from build123d import *

# Parameters (mm, degrees)
SKETCH1_W               = 35
SKETCH1_H               = 25
BOSS_EXTRUDE1_DEPTH     = 8.5
SKETCH3_W               = 32
SKETCH3_H               = 25
CUT_EXTRUDE1_DEPTH      = 7
FILLET1_R               = 1
CHAMFER1_SIZE           = 2.5
SKETCH4_R               = 1.25
CUT_EXTRUDE2_DEPTH      = 35
SKETCH5_R               = 3
BOSS_EXTRUDE3_DEPTH     = 2.5
SKETCH7_R               = 4
SKETCH7_R_2             = 1.25
CUT_EXTRUDE3_DEPTH      = 2.5
CUT_EXTRUDE3_DEPTH_BACK = 1.5


with BuildPart() as part:
    # Sketch1 → Boss-Extrude1 (new body)
    with BuildSketch(Plane.XY):
        with Locations((17.5, 12.5)):
            Rectangle(SKETCH1_W, SKETCH1_H)
    extrude(amount=BOSS_EXTRUDE1_DEPTH)

    # Sketch3 → Cut-Extrude1 (cut)
    with BuildSketch(Plane.XY.offset(8.5)):
        with Locations((17.5, 12.5)):
            Rectangle(SKETCH3_W, SKETCH3_H)
    extrude(amount=-CUT_EXTRUDE1_DEPTH, mode=Mode.SUBTRACT)

    # Fillet1
    fillet1_edges = [part.edges().sort_by_distance(p)[0] for p in [
        (0, 12.5, 0),
        (35, 12.5, 0),
    ]]
    fillet(fillet1_edges, radius=FILLET1_R)

    # Chamfer1
    chamfer1_edges = [part.edges().sort_by_distance(p)[0] for p in [
        (0.75, 0, 8.5),
        (0.75, 25, 8.5),
        (34.25, 0, 8.5),
        (34.25, 25, 8.5),
    ]]
    chamfer(chamfer1_edges, length=CHAMFER1_SIZE)

    # Sketch4 → Cut-Extrude2 (cut)
    with BuildSketch(Plane.ZY):
        with Locations((6, 20)):
            Circle(SKETCH4_R)
        with Locations((6, 4)):
            Circle(SKETCH4_R)
    extrude(amount=-CUT_EXTRUDE2_DEPTH, mode=Mode.SUBTRACT)

    # Sketch5 → Boss-Extrude3 (add)
    with BuildSketch(Plane.XY.offset(1.5)):
        with Locations((9.5, 4.5)):
            Circle(SKETCH5_R)
        with Locations((25.5, 4.5)):
            Circle(SKETCH5_R)
        with Locations((25.499999171, 20.5)):
            Circle(SKETCH5_R)
        with Locations((9.499999171, 20.5)):
            Circle(SKETCH5_R)
    extrude(amount=BOSS_EXTRUDE3_DEPTH)

    # Sketch7 → Cut-Extrude3 (cut, two sides)
    with BuildSketch(Plane.XY.offset(1.5)) as cut_extrude3_sk:
        with Locations((17.5, 12.5)):
            Circle(SKETCH7_R)
        with Locations((9.5, 4.5)):
            Circle(SKETCH7_R_2)
        with Locations((17.5, 4.5)):
            Circle(SKETCH7_R_2)
        with Locations((25.5, 4.5)):
            Circle(SKETCH7_R_2)
        with Locations((25.5, 12.5)):
            Circle(SKETCH7_R_2)
        with Locations((17.5, 20.5)):
            Circle(SKETCH7_R_2)
        with Locations((25.5, 20.5)):
            Circle(SKETCH7_R_2)
        with Locations((9.5, 12.5)):
            Circle(SKETCH7_R_2)
        with Locations((9.5, 20.5)):
            Circle(SKETCH7_R_2)
    extrude(amount=CUT_EXTRUDE3_DEPTH, mode=Mode.SUBTRACT)
    extrude(cut_extrude3_sk.sketch, amount=-CUT_EXTRUDE3_DEPTH_BACK, mode=Mode.SUBTRACT)


solid = part.part
Geometry check sheet. Reference: the model listing, model coordinates, mm. A direction names the side the tool comes from. Coordinates: 2 decimals unless noted, no trailing zeros. Order: outer loops, then holes, each group sorted by start corner. A loop starts at its lowest first (then second) coordinate and runs counter-clockwise, first axis right, second up. Notation, with made-up numbers: (27.25, -29) -> (42.25, -29) arc R25 cw to (42.25, -11) -> close; hole circle Ø5 at (-0.5, 56.5). An arc over 180 degrees is marked (long way). Use a Markdown table: item, result. Add a question column.
1. Go/stop test with flat-tipped pins: pin 1 Ø2 at (y, z) = (20, 6) entering from +X; pin 2 Ø5 at (x, y) = (24.5, 5) entering from +Z; pin 3 Ø3 at (x, y) = (17.5, 4.5) entering from +Z; pin 4 Ø3 at (x, z) = (21.5, 4) entering from +Y. Record where each tip stops, or that it passes through.
2. Cross-section at D-D (y = 9.25). Enter the section's corners in (x, z).
3. Set-up check for faces 5 (the face through (1, 24, 7)), 6 (the face through (28.27, 19.35, 2.73)), 7 (the face through (33.5, 12, 5)): record each of +Z, -Z, +X, -X, +Y, -Y from which the full face is reachable in a straight line by a thin tool's end or side.
4. Cross-section at B-B (x = 9.5). Enter the section's corners in (y, z).
5. Cross-section at C-C (y = 11.75). Enter the section's corners in (x, z), and give its area (3 significant figures).
6. Cross-section at A-A (z = 3.5). Give the number of separate pieces and of enclosed holes in the cut face, and give its area (3 significant figures).
7. Material ranges on L1, parallel to Y at x = 25.5, z = 0.4; L2, parallel to Y at x = 17.5, z = 0.6; L3, parallel to X at y = 2.5, z = 6.75, recorded low to high.
8. Mould release check, pull along X, two halves, no side actions. Record for faces 1 (the face through (27, 5, 4)), 2 (the face through (0.285, 12.675, 0.301)), 3 (the face through (25, 19, 4)), 4 (the face through (34, 24, 7)): pulls with the +X half, pulls with the -X half, needs draft (parallel to the pull), parting line crosses it, or undercut.
Filled sheet:
| question | item | result |
|---|---|---|
| 1 | pin 1 | through |
| 1 | pin 2 | z = 4 |
| 1 | pin 3 | z = 1.5 |
| 1 | pin 4 | y = 22.16 |
| 2 | outline | (0, 1) arc R1 ccw to (1, 0) -> (15.17, 0) -> (15.17, 1.5) -> (1.5, 1.5) -> (1.5, 8.5) -> (0, 8.5) -> close; (19.83, 0) -> (34, 0) arc R1 ccw to (35, 1) -> (35, 8.5) -> (33.5, 8.5) -> (33.5, 1.5) -> (19.83, 1.5) -> close |
| 3 | face 5 | +Z, +X, -X, +Y |
| 3 | face 6 | +Z |
| 3 | face 7 | +Z, +Y, -Y |
| 4 | outline | (0, 0) -> (3.25, 0) -> (3.25, 4) -> (1.5, 4) -> (1.5, 1.5) -> (0, 1.5) -> close; (5.75, 0) -> (11.25, 0) -> (11.25, 1.5) -> (7.5, 1.5) -> (7.5, 4) -> (5.75, 4) -> close; (13.75, 0) -> (19.25, 0) -> (19.25, 4) -> (17.5, 4) -> (17.5, 1.5) -> (13.75, 1.5) -> close; (21.75, 0) -> (25, 0) -> (25, 1.5) -> (23.5, 1.5) -> (23.5, 4) -> (21.75, 4) -> close |
| 5 | outline | (0, 1) arc R1 ccw to (1, 0) -> (8.5, 0) -> (8.5, 1.5) -> (1.5, 1.5) -> (1.5, 8.5) -> (0, 8.5) -> close; (10.5, 0) -> (13.57, 0) -> (13.57, 1.5) -> (10.5, 1.5) -> close; (21.43, 0) -> (24.5, 0) -> (24.5, 1.5) -> (21.43, 1.5) -> close; (26.5, 0) -> (34, 0) arc R1 ccw to (35, 1) -> (35, 8.5) -> (33.5, 8.5) -> (33.5, 1.5) -> (26.5, 1.5) -> close |
| 5 | area | 55.3 mm2 |
| 6 | separate pieces | 6 |
| 6 | enclosed holes | 4 |
| 6 | area | 168 mm2 |
| 7 | L1 | 0 to 3.25, 5.75 to 11.25, 13.75 to 19.25, 21.75 to 25 |
| 7 | L2 | 0 to 3.25, 5.75 to 8.5, 16.5 to 19.25, 21.75 to 25 |
| 7 | L3 | 0 to 1.5, 33.5 to 35 |
| 8 | face 1 | undercut |
| 8 | face 2 | pulls with the -X half |
| 8 | face 3 | undercut |
| 8 | face 4 | needs draft |
